Input: dimensioned drawing with shaded views. Units: mm. Origin: part minimum x, y, z. A direction names the side the tool comes from. Give positions to 0.01 mm unless a question says otherwise; leave off trailing zeros. Write each loop counter-clockwise with the first axis right and the second up, starting at its lowest first coordinate (ties: lowest second). Pieces come first, ordered by that corner, then holes. Notation, with made-up numbers: (-0.75, -19.5) - (35.25, -19.5) arc R16 ccw to (35.25, 9.5) - close; hole circle Ø5 at (59.25, 84). An arc over 180 degrees is marked (long way). Answer as CSV lines item,"result".
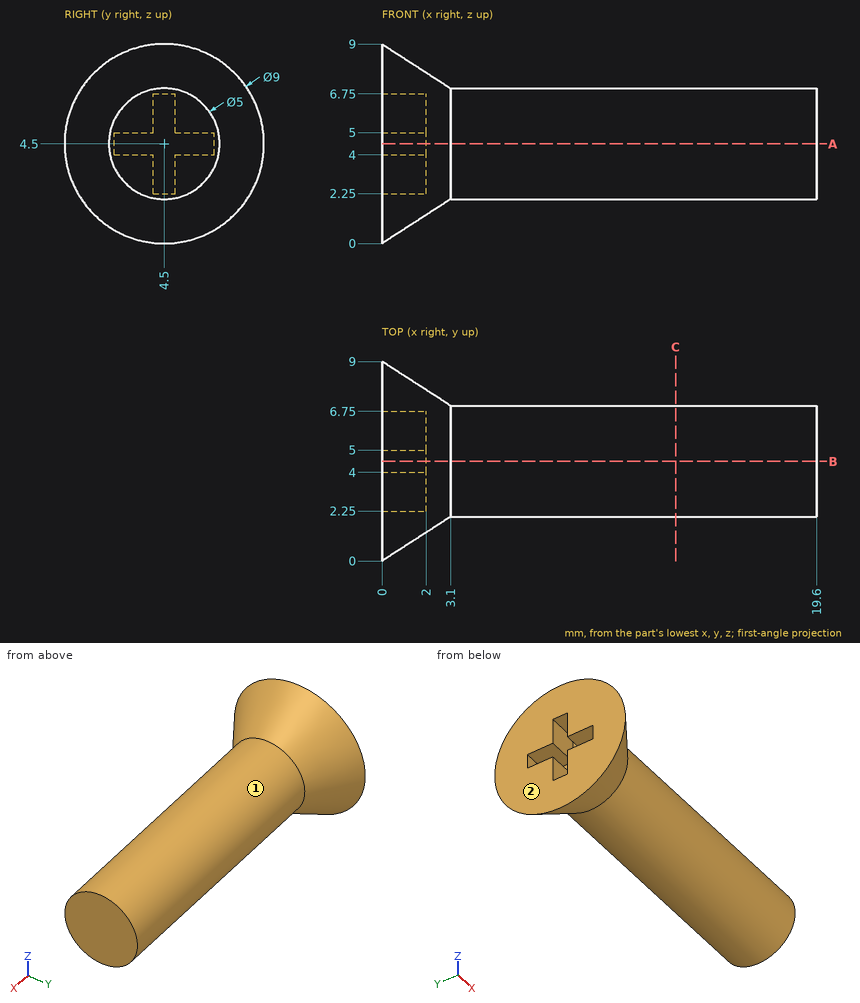
Item 1: Cut plane C-C on x = 13.25. Return the cut outline in (y, z), plus the area to 3 significant figures.
The answers:
outline,"circle Ø5 at (4.5, 4.5)"
area,"19.6 mm²"
Item 2: Contact query for flat-ended pins moving along their axis: pin 1 (0.5 mm diameter, centred on x = 1.5, z = 3, fed in from -Y); pin 2 (2 mm diameter, centred on x = 11, y = 6, fed in from +Z); pin 3 (0.8 mm diameter, centred on x = 1, y = 4.5, fed in from -Z). Output: stop coordinate, or through.
The answers:
pin 1,"y = 1.1"
pin 2,"z = 6.95"
pin 3,"z = 0.39"
Item 3: Ray query, line 1 (Y direction, x = 2.25, z = 6.25); line 2 (X direction, y = 4.25, z = 6); line 3 (X direction, y = 3.5, z = 8.75). Return the intervals inside material, ascending. Write a range as from..to.
The answers:
line 1,"2..7"
line 2,"2..19.6"
line 3,"0..0.21"
Item 4: Reachability of the marked faces 1 and 2 from +Z, -Z, +X, -X, +Y, -Y: full face, straight path, thin tool, end or side. Return the list, or none.
The answers:
face 1,"+X"
face 2,"+Z, -Z, -X, +Y, -Y"
Item 5: Cut plane A-A on z = 4.5. Return the cut outline in (x, y).
The answers:
outline,"(0, 0) - (3.1, 2) - (19.6, 2) - (19.6, 7) - (3.1, 7) - (0, 9) - (0, 6.75) - (2, 6.75) - (2, 2.25) - (0, 2.25) - close"
